```python
from build123d import *

# Parameters (mm, degrees)
F1_DEPTH  = 2
F2_R      = 9.5
F3_DEPTH  = 21
F5_DEPTH  = 16
F6_R      = 0.75
F7_DEPTH  = 14
F8_R      = 0.6
F9_R      = 1.765
F9_R_2    = 1.75
F10_DEPTH = 2
F11_SIZE  = 0.99999


# Not quite as in the source:
# - a fillet or chamfer is up to 0.001 mm smaller than in the source, because OpenCascade refuses the exact size


with BuildPart() as f1:
    # F0 (on Front) → F1 (new body)
    with BuildSketch(Plane.XZ):
        with BuildLine():
            Line((21, 0), (1, 0))
            ThreePointArc((1, 0), (0.2928932188, -0.2928932188), (0, -1))
            Line((0, -1), (0, -36))
            ThreePointArc((0, -36), (0.2928932188, -36.7071067812), (1, -37))
            Line((1, -37), (21, -37))
            ThreePointArc((21, -37), (21.7071067812, -36.7071067812), (22, -36))
            Line((22, -36), (22, -1))
            ThreePointArc((22, -1), (21.7071067812, -0.2928932188), (21, 0))
        make_face()
    extrude(amount=F1_DEPTH)

    # F2 (on face) → F3 (join)
    with BuildSketch(Plane.XZ.offset(2)):
        with Locations((11, -18.5)):
            Circle(F2_R)
    extrude(amount=-F3_DEPTH)

    # F4 (on face) → F5 (cut)
    with BuildSketch(Plane.XZ.offset(2)):
        with BuildLine():
            ThreePointArc((16.5855182065, -12.7726981601), (3.6282924077, -21.6077205753), (19, -18.5))
            ThreePointArc((19, -18.5), (18.5514473986, -15.8588558944), (17.2560894533, -13.5138848036))
            ThreePointArc((17.2560894533, -13.5138848036), (16.561616122, -13.4682581434), (16.5855182065, -12.7726981601))
        make_face()
        with BuildLine():
            ThreePointArc((16.5855182065, -12.7726981601), (16.561616122, -13.4682581434), (17.2560894533, -13.5138848036))
            ThreePointArc((17.2560894533, -13.5138848036), (16.9323905302, -13.1328086863), (16.5855182065, -12.7726981601))
        make_face()
        with BuildLine():
            ThreePointArc((16.5855182065, -12.7726981601), (16.9323905302, -13.1328086863), (17.2560894533, -13.5138848036))
            ThreePointArc((17.2560894533, -13.5138848036), (17.3861798324, -13.3427497952), (17.4323905302, -13.1328086863))
            ThreePointArc((17.4323905302, -13.1328086863), (17.128048188, -12.6726803554), (16.5855182065, -12.7726981601))
        make_face()
    extrude(amount=-F5_DEPTH, mode=Mode.SUBTRACT)

    # F6 (on face) → F7 (join)
    with BuildSketch(Plane.XZ.offset(-14)):
        with Locations((14.4535416495, -22.7805431986)):
            Circle(F6_R)
        with Locations((8.4928393267, -23.3953187188)):
            Circle(F6_R)
        with Locations((5.5545138952, -19.272451346)):
            Circle(F6_R)
        with Locations((16.4460298856, -17.7313918519)):
            Circle(F6_R)
    extrude(amount=F7_DEPTH)

    # F8
    f8_edges = [f1.edges().sort_by_distance(p)[0] for p in [
        (15.69603, 0, -17.731392),
        (13.703542, 0, -22.780543),
        (7.742839, 0, -23.395319),
        (4.804514, 0, -19.272451),
    ]]
    fillet(f8_edges, radius=F8_R)

    # F9 (on face) → F10 (cut, through all)
    with BuildSketch(Plane.XZ.offset(2)):
        with Locations((11, -32)):
            Circle(F9_R)
        with Locations((11, -5)):
            Circle(F9_R_2)
    extrude(amount=-F10_DEPTH, mode=Mode.SUBTRACT)

    # F11 (size 1 in the source; OpenCascade refuses exactly that, so slightly less here)
    f11_edges = [f1.edges().sort_by_distance(p)[0] for p in [
        (9.25, -2, -5),
        (9.235, -2, -32),
        (22, -2, -18.5),
        (11, -2, -37),
        (0, -2, -18.5),
        (11, -2, 0),
        (21.707107, -2, -0.292893),
        (0.292893, -2, -0.292893),
        (21.707107, -2, -36.707107),
        (0.292893, -2, -36.707107),
    ]]
    chamfer(f11_edges, length=F11_SIZE)


solid = f1.part
```
CAD build for the part. Positions are in the model's coordinates, mm. A direction names the side the tool comes from. Coordinates: 2 decimals unless noted, no trailing zeros. Order: outer loops, then holes, each group sorted by start corner. A loop starts at its lowest first (then second) coordinate and runs counter-clockwise, first axis right, second up. Notation, with made-up numbers: M -26,23.5 L 13,23.5 A27 ccw 13,47.5 Z; hole C 0,-19 d7. An arc over 180 degrees is marked long. Answer as CSV lines item,"result".
1) Mould opens along X. For faces 4 (the cylindrical face through (5, 7.39, -18.77)), 5 (the cylindrical face through (12.617, -0.507, -5.67)), 6 (the flat face through (22, -0.5, -18.7)), 7 (the flat face through (6, 0, -10)) say: released by +X, released by -X, zero draft, split by the parting line, or undercut.
Verdict:
face 4,"undercut"
face 5,"undercut"
face 6,"released by +X"
face 7,"zero draft"
2) Cut at B-B (z = -32). List the corners of the cut face in (x, y) (3 decimals).
Verdict:
outline,"M 0,-1 L 1,-2 L 8.235,-2 L 9.235,-1 L 9.235,0 L 0,0 Z; M 12.765,-1 L 13.765,-2 L 21,-2 L 22,-1 L 22,0 L 12.765,0 Z"
3) 3-axis set-ups, long thin cutter, end or side, ignore diameter. For faces 1 (the cylindrical face through (19.776, 9.367, -22.139)), 2 (the flat face through (11, 19, -18)), 3 (the flat face through (11, 14, -18)): which of +Z, -Z, +X, -X, +Y, -Y reach the whole face in a straight line?
Verdict:
face 1,"+Y"
face 2,"+Z, -Z, +X, -X, +Y"
face 3,"-Y"
4) Cut at A-A (x = 11). List the corners of the cut face in (y, z) (3 decimals), then the cut area to 3 significant figures.
Verdict:
outline,"M -2,-36 L -1,-37 L 0,-37 L 0,-33.765 L -1,-33.765 L -2,-34.765 Z; M -2,-29.235 L -1,-30.235 L 0,-30.235 L 0,-28 L 19,-28 L 19,-9 L 0,-9 L 0,-6.75 L -1,-6.75 L -2,-7.75 L -2,-10.5 L 14,-10.5 L 14,-26.5 L -2,-26.5 Z; M -2,-2.25 L -1,-3.25 L 0,-3.25 L 0,0 L -1,0 L -2,-1 Z"
area,"162 mm2"
5) Drill centre lines: L1, parallel to Z at x = 11, y = -0.25 (3 decimals); L2, parallel to X at y = 7.75, z = -18; L3, parallel to Z at x = 11, y = 6.25. Where is each one in solid material? Low to high. Write a range as from..to.
Verdict:
L1,"-37..-33.765, -30.235..-26.5, -10.5..-6.75, -3.25..0"
L2,"1.51..3.02, 15.75..17.15, 18.98..20.49"
L3,"-28..-26.5, -10.5..-9"
6) Cut at C-C (y = 13.25). List the corners of the cut face in (x, z).
Verdict:
outline,"C 11,-18.5 d19; C 5.55,-19.27 d1.5; C 8.49,-23.4 d1.5; C 14.45,-22.78 d1.5; C 16.45,-17.73 d1.5; hole M 16.59,-12.77 A8 ccw long 17.26,-13.51 A0.5 ccw long Z"
7) Flat gauge pins, fed straight in: P1, Ø4, axis at y = 8, z = -12.5, coming from the -X side; P2, Ø8, axis at x = 9, z = -21.5, coming from the -Y side; P3, Ø1.5, axis at y = 15.5, z = -9.5, coming from the -X side. Where does each tip first touch, or does it go through?
Verdict:
P1,"x = 2.38"
P2,"y = 0"
P3,"x = 6.29"
8) Cut at D-D (z = -21.5). List the corners of the cut face in (x, y), then the cut area to 3 significant figures.
Verdict:
outline,"M 0,-1 L 1,-2 L 3.58,-2 L 3.58,14 L 18.42,14 L 18.42,-2 L 21,-2 L 22,-1 L 22,0 L 20.01,0 L 20.01,19 L 1.99,19 L 1.99,0 L 0,0 Z"
area,"148 mm2"
